The figure shows three views and two pictorial views of one solid part (mm, origin at its lowest corner). Answer the questions. A direction names the side the tool comes from. Round coordinates to 2 decimals unless told otherwise and drop trailing zeros. Write each loop counter-clockwise with the first axis right and the second up, starting at its lowest first coordinate (ties: lowest second). Pieces come first, ordered by that corner, then holes.
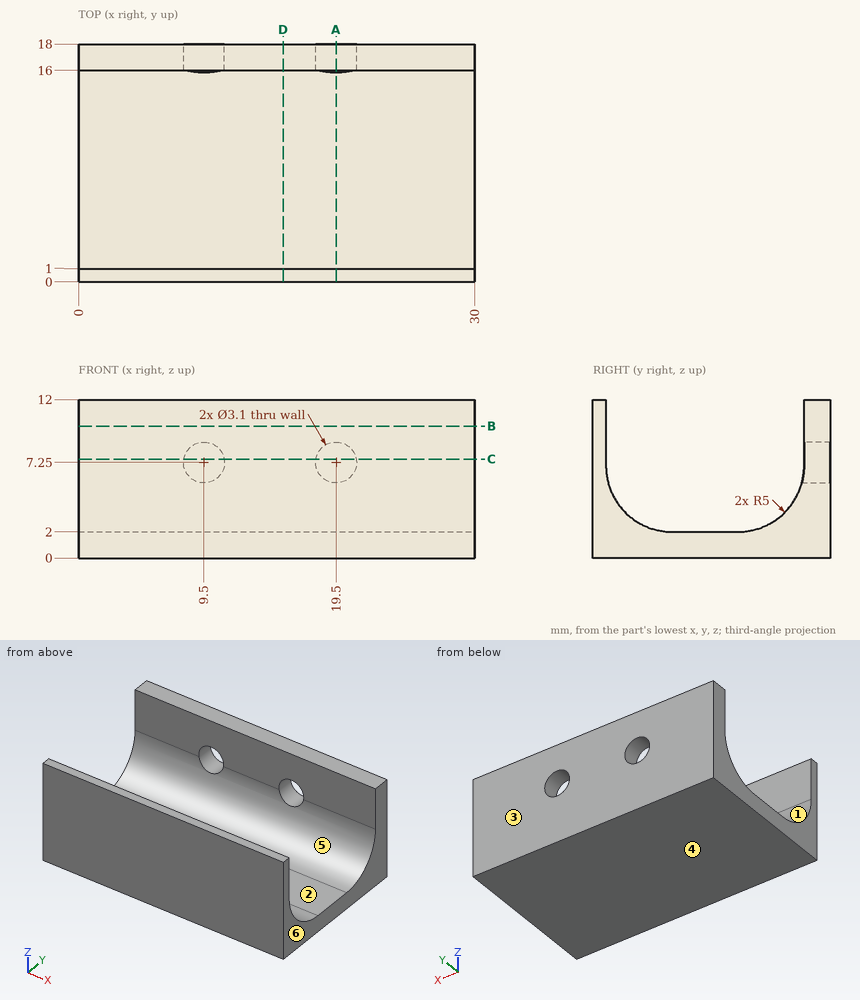
Q1. Straight lines are drawn through the part: probe 1 along X at (y, z) = (17.3, 7.25); probe 2 along Y at (x, z) = (4, 8.75); probe 3 along Z at (x, y) = (7.5, 11.25). For each, find the intervals that lie inside material, in ascending order.
Verdict:
probe 1: x = 0 to 7.95, 11.05 to 17.95, 21.05 to 30
probe 2: y = 0 to 1, 16 to 18
probe 3: z = 0 to 2.01
Q2. Flat-ended cylindrical pins translate along their axes: pin 1 Ø5.5 at (x, y) = (14, 9) entering from +Z; pin 2 Ø4 at (x, y) = (6, 11) entering from +Z; pin 3 Ø3 at (x, y) = (19.5, 11) entering from +Z. Find the tip coordinate at first contact, or state that the pin passes through.
Verdict:
pin 1: stops at z = 2.06
pin 2: stops at z = 2.42
pin 3: stops at z = 2.23
Q3. Section C-C (z = 7.5) is taken. Determine the outline of the cut face in (x, y), then the cut area to 3 significant figures.
Verdict:
outline: (0, 0) - (30, 0) - (30, 1) - (0, 1) - close; (0, 16) - (7.97, 16) - (7.97, 18) - (0, 18) - close; (11.03, 16) - (17.97, 16) - (17.97, 18) - (11.03, 18) - close; (21.03, 16) - (30, 16) - (30, 18) - (21.03, 18) - close
area: 77.8 mm2
Q4. Which of the six approach directions +Z, -Z, +X, -X, +Y, -Y give full straight-line access (tool end or side, diameter ignored) to the marked faces 5 and 6?
Verdict:
face 5: +Z, +X, -X
face 6: +Z, -Z, +X, +Y, -Y
Q5. Determine the mould class of the marked faces 1, 2, 3 and 4 for opening direction Y: pulls with the +Y half, pulls with the -Y half, needs draft (parallel to the pull), parting line crosses it, or undercut.
Verdict:
face 1: undercut
face 2: undercut
face 3: pulls with the +Y half
face 4: needs draft
Q6. Section B-B (z = 10) is taken. Determine the outline of the cut face in (x, y), then the cut area to 3 significant figures.
Verdict:
outline: (0, 0) - (30, 0) - (30, 1) - (0, 1) - close; (0, 16) - (30, 16) - (30, 18) - (0, 18) - close
area: 90.0 mm2
Q7. Section A-A (x = 19.5) is taken. Determine the outline of the cut face in (y, z), then the cut area to 3 significant figures.
Verdict:
outline: (0, 0) - (18, 0) - (18, 5.7) - (15.83, 5.7) arc R5 cw to (11, 2) - (6, 2) arc R5 cw to (1, 7) - (1, 12) - (0, 12) - close; (16, 8.8) - (18, 8.8) - (18, 12) - (16, 12) - close
area: 70.5 mm2
Q8. Section D-D (x = 15.5) is taken. Determine the outline of the cut face in (y, z), then the cut area to 3 significant figures.
Verdict:
outline: (0, 0) - (18, 0) - (18, 12) - (16, 12) - (16, 7) arc R5 cw to (11, 2) - (6, 2) arc R5 cw to (1, 7) - (1, 12) - (0, 12) - close
area: 76.7 mm2
